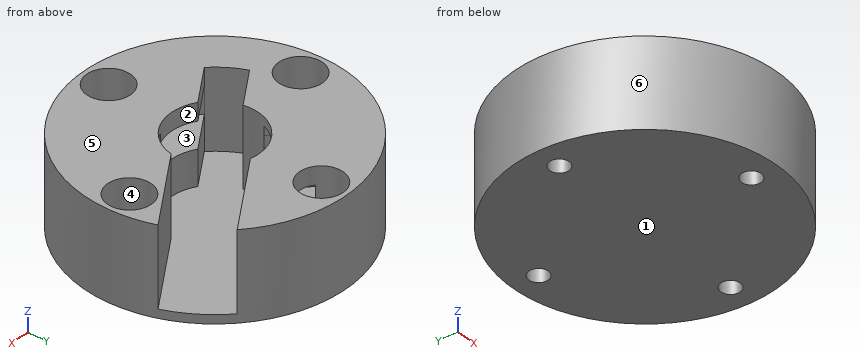
from build123d import *

# Parameters (mm, degrees)
SKETCH1_R                = 15
BOSS_EXTRUDE1_DEPTH      = 10
SKETCH1_3_R              = 1.1
SCREWTHREAD_CUTOUT_DEPTH = 24.452078799
SCREW_START              = 4
SKETCH1_4_R              = 2.5
SCREW_HEAD_CUTOUT_DEPTH  = 20.452078799
CIRPATTERN1_COUNT        = 4
CUT_EXTRUDE3_START       = 1
CUT_EXTRUDE3_DEPTH       = 23.452078799
CUT_EXTRUDE4_START       = 5
CUT_EXTRUDE4_DEPTH       = 3
CUT_EXTRUDE11_START      = 1
CUT_EXTRUDE11_DEPTH      = 8


with BuildPart() as part:
    # Sketch1 → Boss-Extrude1 (new body)
    with BuildSketch(Plane.XY):
        Circle(SKETCH1_R)
    extrude(amount=BOSS_EXTRUDE1_DEPTH)

    # Sketch1_3 → screwthread cutout (cut, through all)
    with BuildSketch(Plane.XY):
        with Locations((12, 0)):
            Circle(SKETCH1_3_R)
    screwthread_cutout = extrude(amount=SCREWTHREAD_CUTOUT_DEPTH, mode=Mode.SUBTRACT)

    # Sketch1_4 → screw head cutout (cut, through all)
    with BuildSketch(Plane.XY.offset(SCREW_START)):
        with Locations((12, 0)):
            Circle(SKETCH1_4_R)
    screw_head_cutout = extrude(amount=SCREW_HEAD_CUTOUT_DEPTH, mode=Mode.SUBTRACT)

    # CirPattern1: screwthread cutout, screw head cutout ×4 about axis
    cirpattern1_axis = Axis((0, 0, 0), (0, 0, 1))
    add([screwthread_cutout.rotate(cirpattern1_axis, i * 360 / CIRPATTERN1_COUNT) for i in range(1, CIRPATTERN1_COUNT)], mode=Mode.SUBTRACT)
    add([screw_head_cutout.rotate(cirpattern1_axis, i * 360 / CIRPATTERN1_COUNT) for i in range(1, CIRPATTERN1_COUNT)], mode=Mode.SUBTRACT)

    # Sketch2 → Cut-Extrude3 (cut, through all)
    with BuildSketch(Plane.XY.offset(CUT_EXTRUDE3_START)):
        with BuildLine():
            Line((14.925030647, 5.453756521), (11.13336398, 11.337910146))
            Line((11.13336398, 11.337910146), (1.105685379, 4.876213679))
            ThreePointArc((1.105685379, 4.876213679), (-3.424108155, 3.643553669), (-4.935416103, -0.801041751))
            Line((-4.935416103, -0.801041751), (-9.489267084, -3.735479917))
            ThreePointArc((-9.489267084, -3.735479917), (-8.572404045, -5.523937806), (-7.322600417, -7.097853417))
            Line((-7.322600417, -7.097853417), (-2.768749437, -4.163415252))
            ThreePointArc((-2.768749437, -4.163415252), (1.903153532, -4.623635651), (4.897352046, -1.007939947))
            Line((4.897352046, -1.007939947), (14.925030647, 5.453756521))
        make_face()
    extrude(amount=CUT_EXTRUDE3_DEPTH, mode=Mode.SUBTRACT)

    # Sketch2_4 → Cut-Extrude4 (cut)
    with BuildSketch(Plane.XY.offset(CUT_EXTRUDE4_START)):
        with BuildLine():
            ThreePointArc((-7.322600417, -7.097853417), (-1.050685684, -10.143769496), (5.712369236, -8.448007914))
            Line((5.712369236, -8.448007914), (8.522190031, -5.601096061))
            Line((8.522190031, -5.601096061), (4.666457664, -1.795598194))
            ThreePointArc((4.666457664, -1.795598194), (1.517222308, -4.764245635), (-2.768749437, -4.163415252))
            Line((-2.768749437, -4.163415252), (-7.322600417, -7.097853417))
        make_face()
        with BuildLine():
            Line((-5.712369236, 8.448007914), (-8.522190031, 5.601096061))
            Line((-8.522190031, 5.601096061), (-4.666457664, 1.795598194))
            ThreePointArc((-4.666457664, 1.795598194), (-2.35421383, 4.411085722), (1.105685379, 4.876213679))
            Line((1.105685379, 4.876213679), (6.155892888, 8.130497079))
            ThreePointArc((6.155892888, 8.130497079), (0.272729885, 10.194391517), (-5.712369236, 8.448007914))
        make_face()
    extrude(amount=CUT_EXTRUDE4_DEPTH, mode=Mode.SUBTRACT)

    # Sketch2_5 → Cut-Extrude11 (cut)
    with BuildSketch(Plane.XY.offset(CUT_EXTRUDE11_START)):
        Polygon((5.712369236, -8.448007914), (-8.522190031, 5.601096061), (-5.712369236, 8.448007914), (8.522190031, -5.601096061), align=None)
    extrude(amount=CUT_EXTRUDE11_DEPTH, mode=Mode.SUBTRACT)


solid = part.part
Check sheet for the modelled part. Datum: model origin and axes. Units: mm. Face numbers are marked on the shaded views. A direction names the side the tool comes from. Round coordinates to 2 decimals unless told otherwise and drop trailing zeros. Order: outer loops, then holes, each group sorted by start corner. A loop starts at its lowest first (then second) coordinate and runs counter-clockwise, first axis right, second up. Notation, with made-up numbers: M 36,-25 L 56,-25 A26 ccw 56,6 Z; hole C -32.75,51 d1. An arc over 180 degrees is marked long. One line per item, written item: value. Start each with the question number.
1. Section check B-B on x = 0. Give the number of separate pieces and of enclosed holes in the cut face, and give its area (3 significant figures).
2. Section check D-D on z = 7. Enter the section's corners in (x, y).
3. Access from +Z, -Z, +X, -X, +Y, -Y to the whole of each face (thin tool, end or side, straight path). Record for the marked faces 1, 2 and 3.
4. Section check A-A on y = -12. Enter the section's corners in (x, z).
5. Release check for a two-part mould opening along Y. For the marked faces 4, 5 and 6 record: released by +Y, released by -Y, zero draft, split by the parting line, or undercut.
6. Scan lines: line 1 along Z through (x, y) = (1.75, 7.25); line 2 along Y through (x, z) = (5.75, 7.25); line 3 along X through (y, z) = (0.5, 5.25). Record each from-to range of solid material in increasing order.
7. Gauge pin test, flat ends, axial feed: P1, Ø1.5, axis at x = 12, z = 2.5, coming from the -Y side; P2, Ø4, axis at x = 0, y = 12, coming from the +Z side; P3, Ø1, axis at x = 8, z = 6.5, coming from the +Y side. Record the tip position at first contact, or that the pin passes through.
8. Section check C-C on z = 2.75. Enter the section's corners in (x, y), and give its area (3 significant figures).
Results found:
1. separate pieces: 5
1. enclosed holes: 0
1. area: 105 mm^2
2. outline: M -9.49,-3.74 L -4.94,-0.8 A5 cw -4.67,1.8 L -8.52,5.6 L -5.71,8.45 A10.2 cw -1.59,10.07 A2.5 cw long 1.59,10.07 A10.2 cw 6.16,8.13 L 10.37,10.84 A15 ccw long 14.16,4.96 L 4.9,-1.01 A5 cw 4.67,-1.8 L 8.52,-5.6 L 5.71,-8.45 A10.2 cw 1.59,-10.07 A2.5 cw long -1.59,-10.07 A10.2 cw Z; hole C -12,0 d5; hole C 12,0 d5
3. face 1: -Z, +X, -X, +Y, -Y
3. face 2: +Z
3. face 3: none
4. outline: M -9,0 L -1.1,0 L -1.1,4 L -2.5,4 L -2.5,10 L -9,10 Z; M 1.1,0 L 9,0 L 9,10 L 2.5,10 L 2.5,4 L 1.1,4 Z
5. face 4: undercut
5. face 5: zero draft
5. face 6: split by the parting line
6. line 1: 0 to 5, 8 to 10
6. line 2: -13.85 to -8.41, -2.87 to -0.46, 8.42 to 13.85
6. line 3: -14.99 to -14.45, -9.55 to -4.97, 7.24 to 9.55, 14.45 to 14.99
7. P1: y = -9.92
7. P2: z = 4
7. P3: y = 12.99
8. outline: M -9.49,-3.74 L -4.94,-0.8 A5 cw -4.67,1.8 L -8.52,5.6 L -5.71,8.45 L -1.86,4.64 A5 cw 1.11,4.88 L 10.37,10.84 A15 ccw long 14.16,4.96 L 4.9,-1.01 A5 cw 4.67,-1.8 L 8.52,-5.6 L 5.71,-8.45 L 1.86,-4.64 A5 cw -2.77,-4.16 L -7.32,-7.1 A10.2 cw Z; hole C -12,0 d2.2; hole C 0,-12 d2.2; hole C 0,12 d2.2; hole C 12,0 d2.2
8. area: 479 mm^2
